Input: part model. Units: mm. Frame: model coordinates. Face numbers are marked on the shaded views. A direction names the side the tool comes from. Round coordinates to 2 decimals unless told otherwise and drop trailing zeros. Write each loop counter-clockwise with the first axis right and the second up, starting at its lowest first coordinate (ties: lowest second). Pieces come first, ordered by that corner, then holes. Notation, with made-up numbers: (71, -12) -> (92, -12) arc R14 ccw to (92, 10) -> close; hole circle Ø10 at (20, 35.5). An arc over 180 degrees is marked (long way). Write item = value, one per line. Start each with the question number.
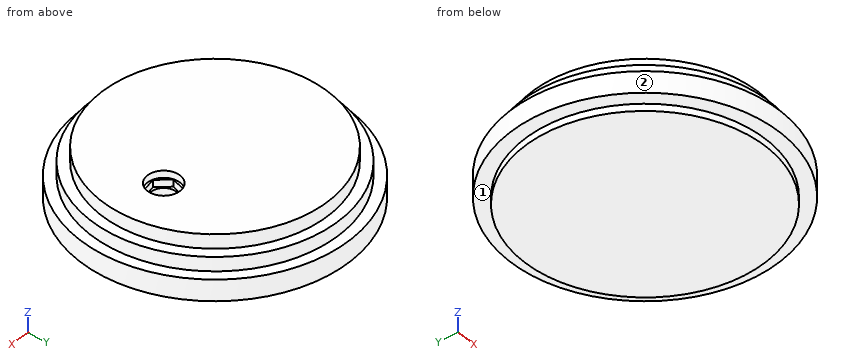
```python
from build123d import *

# Parameters (mm, degrees)
F2_R     = 1.75
F3_DEPTH = 7
F4_R     = 1.75
F5_DEPTH = 2
F6_R     = 2.3
F7_DEPTH = 1


with BuildPart() as f1:
    # F0 (on Front) → F1 (revolve)
    with BuildSketch(Plane.XZ):
        Polygon((0, 8), (0, 0), (17, 0), (17, 1), (19, 1), (19, 4), (17.5, 4), (17.5, 6), (16, 6), (16, 8), align=None)
    revolve(axis=Axis((0, 0, 4), (0, 0, 1)))

    # F2 (on face) → F3 (cut)
    with BuildSketch(Plane.XY.offset(8)):
        with Locations((8.75, 0)):
            Circle(F2_R)
    extrude(amount=-F3_DEPTH, mode=Mode.SUBTRACT)

    # F4 (on face) → F5 (cut)
    with BuildSketch(Plane.XY.offset(8)):
        with Locations((8.75, 0)):
            Circle(F4_R)
        Polygon((10.258503366, -1.66940636), (10.95, 0.4716990566), (9.441496634, 2.1411054166), (7.241496634, 1.66940636), (6.55, -0.4716990566), (8.058503366, -2.1411054166), align=None)
    extrude(amount=-F5_DEPTH, mode=Mode.SUBTRACT)

    # F6 (on face) → F7 (cut)
    with BuildSketch(Plane.XY.offset(8)):
        with Locations((8.75, 0)):
            Circle(F6_R)
    extrude(amount=-F7_DEPTH, mode=Mode.SUBTRACT)


solid = f1.part
```
1. Section C-C (z = 4.5). Output: boundary loops of the cut face in (x, y), then the cut area to 3 significant figures.
2. Reachability of the marked faces 1 and 2 from +Z, -Z, +X, -X, +Y, -Y: full face, straight path, thin tool, end or side. Return the list, or none.
3. Section A-A (x = 0). Output: boundary loops of the cut face in (y, z).
4. Pin query (flat end, axial travel): P1, Ø1.5, axis at x = 7.5, z = 5.5, coming from the +Y side; P2, Ø4.5, axis at x = 8.75, y = 0, coming from the +Z side; P3, Ø3, axis at x = 2.5, z = 3, coming from the -Y side. Return the tip coordinate at first contact, or that it passes through.
5. Section D-D (x = -7.5). Output: boundary loops of the cut face in (y, z).
6. Section B-B (y = 0). Output: boundary loops of the cut face in (x, z).
7. Line query: line 1 along Z through (x, y) = (-15, 9.5); line 2 along Y through (x, z) = (8.75, 2.25); line 3 along Y through (x, z) = (8.75, 7.35). Output: solid intervals per line, ascending.
Check sheet entries:
q1.outline = circle Ø35 at (0, 0); hole circle Ø3.5 at (8.75, 0)
q1.area = 952 mm2
q2.face_1 = -Z
q2.face_2 = +Z, -Z
q3.outline = (-19, 1) -> (-17, 1) -> (-17, 0) -> (17, 0) -> (17, 1) -> (19, 1) -> (19, 4) -> (17.5, 4) -> (17.5, 6) -> (16, 6) -> (16, 8) -> (-16, 8) -> (-16, 6) -> (-17.5, 6) -> (-17.5, 4) -> (-19, 4) -> close
q4.P1 = 16.15
q4.P2 = 7
q4.P3 = -18.97
q5.outline = (-17.46, 1) -> (-15.26, 1) -> (-15.26, 0) -> (15.26, 0) -> (15.26, 1) -> (17.46, 1) -> (17.46, 4) -> (15.81, 4) -> (15.81, 6) -> (14.13, 6) -> (14.13, 8) -> (-14.13, 8) -> (-14.13, 6) -> (-15.81, 6) -> (-15.81, 4) -> (-17.46, 4) -> close
q6.outline = (-19, 1) -> (-17, 1) -> (-17, 0) -> (17, 0) -> (17, 1) -> (19, 1) -> (19, 4) -> (17.5, 4) -> (17.5, 6) -> (16, 6) -> (16, 8) -> (11.05, 8) -> (11.05, 7) -> (10.8, 7) -> (10.8, 6) -> (10.5, 6) -> (10.5, 1) -> (7, 1) -> (7, 6) -> (6.7, 6) -> (6.7, 7) -> (6.45, 7) -> (6.45, 8) -> (-16, 8) -> (-16, 6) -> (-17.5, 6) -> (-17.5, 4) -> (-19, 4) -> close
q7.line_1 = 1 to 4
q7.line_2 = -16.87 to -1.75, 1.75 to 16.87
q7.line_3 = -13.4 to -2.3, 2.3 to 13.4
